```python
from build123d import *

# Parameters (mm, degrees)
SKETCH2_R = 2


with BuildPart() as part:
    # Sketch1 → Cup (revolve)
    with BuildSketch(Plane(origin=(0, 0, 0), x_dir=(-1, 0, 0), z_dir=(0, 1, 0)), mode=Mode.PRIVATE) as cup_sk:
        Polygon((0, 3), (-27.6, 3), (-27.6, 0), (-29.573, 0), (-44.616104, 110.4), (-42.635368, 110.4), (-28.23035, 5), (0, 5), align=None)
    revolve(cup_sk.sketch.rotate(Axis((0, 0, -50), (0, 0, 1)), 180), axis=Axis((0, 0, -50), (0, 0, 1)))

    # Sketch2 → BeadRound (revolve)
    with BuildSketch(Plane(origin=(0, 0, 0), x_dir=(-1, 0, 0), z_dir=(0, 1, 0))):
        with Locations((-45, 110.4)):
            Circle(SKETCH2_R)
    revolve(axis=Axis((0, 0, -50), (0, 0, 1)))


solid = part.part
```
Could you check a few things on this model? Use its own coordinates, in mm. A direction names the side the tool comes from. Round coordinates to 2 decimals unless told otherwise and drop trailing zeros. Write each loop counter-clockwise with the first axis right and the second up, starting at its lowest first coordinate (ties: lowest second). Pieces come first, ordered by that corner, then holes.
(1) Suppose I cut it at C-C on z = 60.5. Write out the boundary of the cut face in (x, y), and give its area (3 significant figures).
Findings below:
outline: circle Ø75.63 at (0, 0); hole circle Ø71.63 at (0, 0)
area: 463 mm2
(2) Suppose I cut it at A-A on x = 0. Write out the boundary of the cut face in (y, z).
Findings below:
outline: (-44.36, 108.51) - (-29.57, 0) - (-27.6, 0) - (-27.6, 3) - (27.6, 3) - (27.6, 0) - (29.57, 0) - (44.36, 108.51) arc R2 ccw (long way) to (43, 110.4) - (42.64, 110.4) - (28.23, 5) - (-28.23, 5) - (-42.64, 110.4) - (-43, 110.4) arc R2 ccw (long way) to start
(3) If I drill on probe 1 along X at (y, z) = (-8, 44.5); probe 2 along Z at (x, y) = (40, -21); probe 3 along X at (y, z) = (16, 77.5), over which ranges is the centre line in solid material (lowest first)?
Findings below:
probe 1: x = -34.73 to -32.66, 32.66 to 34.73
probe 2: z = 108.41 to 112.39
probe 3: x = -36.81 to -34.62, 34.62 to 36.81
(4) For pin 1 (1.5 mm diameter, centred on y = 17, z = 67.5, fed in from -X); pin 2 (6 mm diameter, centred on x = 16.5, z = 33, fed in from -Y); pin 3 (4 mm diameter, centred on y = -14.5, z = 57.5, fed in from -X); pin 4 (8 mm diameter, centred on x = 14, y = 23.5, fed in from -Z), each with a flat end and sliding along its axis, tell me the tip position at first contact or that it passes through.
Findings below:
pin 1: stops at x = -35.22
pin 2: stops at y = -31.35
pin 3: stops at x = -35.31
pin 4: stops at z = 0
(5) Which directions (+Z, -Z, +X, -X, +Y, -Y) give clear straight access to the entire face, cutting with the end or side of a thin tool? Please do faces 1 (the face through (38.4, 18.9, 110.4)), 2 (the face through (29.417, 22.556, 55.012)).
Findings below:
face 1: +Z
face 2: -Z
(6) Suppose I cut it at D-D on z = 37. Write out the boundary of the cut face in (x, y).
Findings below:
outline: circle Ø69.23 at (0, 0); hole circle Ø65.21 at (0, 0)
(7) Thinking about a two-plate mould opening in X: for faces 3 (the face through (20.3, -18.7, 1.5)), 4 (the face through (20, 20, 0)), 5 (the face through (0, 0, 3)), which applies, +X half, -X half, draft (parallel to the pull), parting line (faces both ways), or undercut?
Findings below:
face 3: undercut
face 4: draft
face 5: undercut
